Verification items for the finished model (mm, model axes). Face numbers are marked on the shaded views. A direction names the side the tool comes from. Give positions to 0.01 mm unless a question says otherwise; leave off trailing zeros. Loops run counter-clockwise (first coordinate to the right, second up) from the corner with the lowest first, then second, coordinate; pieces in that order, holes last. Notation, with made-up numbers: M 18,75.25 L 28,75.25 A19 ccw 28,85.25 Z; hole C 88,-10 d1. An arc over 180 degrees is marked long. Answer in a Markdown table with one row per item.
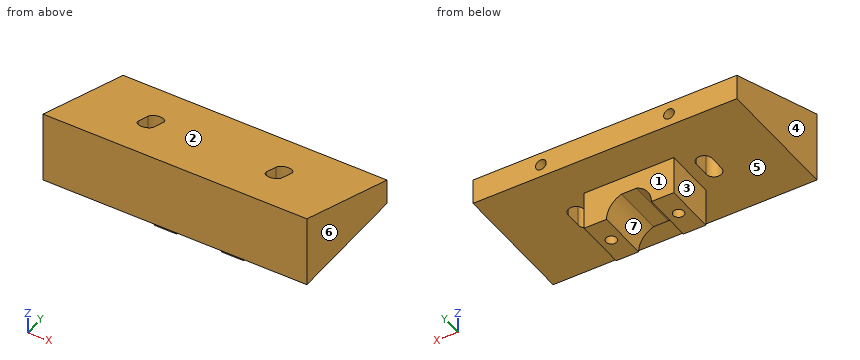
Autodesk Inventor part; units mm, degrees
ref_plane "YZ Plane" through (0, 0, 0) normal (1, 0, 0) x (0, 1, 0)
ref_plane "XZ Plane" through (0, 0, 0) normal (0, 1, 0) x (-1, 0, 0)
ref_plane "XY Plane" through (0, 0, 0) normal (0, 0, 1) x (1, 0, 0)
sketch "Skizze1" plane through (0, 0, 0) normal (0, 1, 0) x (-1, 0, 0)
  line L0 (0, 0) -> (-206, 0)
  line L1 (-206, 0) -> (-206, -20)
  line L2 (-206, -20) -> (0, -20)
  line L3 (0, -20) -> (0, 0)
  dimension "d0" = 206
  dimension "d1" = 20
extrude "Extrusion1" add sketch "Skizze1" against normal blind 100
sketch "Skizze2" plane through (0, 0, 0) normal (0, 1, 0) x (1, 0, 0)
  line L0 (0, 0) -> (0, 10) construction
  line L1 (0, 10) -> (206, 10) construction
  line L2 (0, 10) -> (103, 10) construction
  line L3 (103, 10) -> (53, 10) construction
  line L4 (53, 10) -> (153, 10) construction
  dimension "d4" = 10
  dimension "d5" = 206
  dimension "d6" = 90
  dimension "d7" = 103
  dimension "d8" = 50
  dimension "d9" = 100
hole "Bohrung1" at (153, 0, -10) at (53, 0, -10) direction (0, -1, 0) diameter 8.376 depth 27.3 tip angle 118
sketch "Skizze3" plane through (206, 0, 0) normal (1, 0, 0) x (0, 0, -1)
  line L0 (0, 0) -> (-41.0424, -112.7631)
  line L1 (0, 0) -> (120, 0) construction
  line L2 (0, 0) -> (0, -100)
  line L3 (0, -100) -> (-50, -100)
  line L4 (0, -100) -> (50, -100) construction
  point P0 (-36.397, -100)
  dimension "d17" = 120
  dimension "d18" = 110
  dimension "d19" = 50
  dimension "d20" = 180
extrude "Extrusion2" add sketch "Skizze3" against normal blind 206
sketch "Skizze4" plane through (206, 0, -20) normal (0, 0, -1) x (-1, 0, 0)
  line L0 (206, 0) -> (103, 0) construction
  line L1 (206, 0) -> (309, 0) construction
  line L2 (103, 0) -> (153, 0) construction
  line L3 (0, 0) -> (206, 0) construction
  line L4 (153, 0) -> (53, 0) construction
  line L5 (53, 0) -> (53, -50) construction
  line L6 (53, 0) -> (103, 0) construction
  line L7 (153, 0) -> (153, -50) construction
  line L8 (153, 0) -> (203, 0) construction
  line L9 (53, -50) -> (59, -50)
  line L10 (59, -50) -> (59, -44)
  arc A0 (59, -44) -> (47, -44) centre (53, -44) ccw
  line L11 (53, -44) -> (47, -44) construction
  line L12 (53, -44) -> (59, -44) construction
  line L13 (47, -44) -> (47, -50)
  line L14 (47, -50) -> (59, -50) construction
  line L15 (53, -100) -> (53, -50) construction
  line L16 (59, -50) -> (59, -56)
  arc A1 (47, -56) -> (59, -56) centre (53, -56) ccw
  line L17 (53, -56) -> (47, -56) construction
  line L18 (53, -56) -> (59, -56) construction
  line L19 (47, -56) -> (47, -50)
  line L20 (103, 0) -> (103, -100) construction
  line L21 (103, 0) -> (203, 0) construction
  line L22 (153, -50) -> (147, -50)
  line L23 (147, -50) -> (147, -44)
  arc A2 (159, -44) -> (147, -44) centre (153, -44) ccw
  line L24 (153, -44) -> (159, -44) construction
  line L25 (153, -44) -> (147, -44) construction
  line L26 (159, -44) -> (159, -50)
  line L27 (159, -50) -> (147, -50) construction
  line L28 (147, -50) -> (147, -56)
  line L29 (153, -56) -> (147, -56) construction
  line L30 (153, -56) -> (159, -56) construction
  line L31 (159, -56) -> (159, -50)
  arc A3 (147, -56) -> (159, -56) centre (153, -56) ccw
  dimension "d23" = 103
  dimension "d24" = 180
  dimension "d25" = 50
  dimension "d26" = 100
  dimension "d27" = 0
  dimension "d28" = 50
  dimension "d29" = 90
  dimension "d30" = 50
  dimension "d31" = 90
  dimension "d32" = 6
  dimension "d33" = 6
  dimension "d34" = 180
  dimension "d35" = 100
  dimension "d36" = 90
extrude "Extrusion3" cut sketch "Skizze4" against normal blind 100
sketch "Skizze5" plane through (206, 0, -20) normal (0, 0, -1) x (-1, 0, 0)
  line L0 (206, 0) -> (0, 0)
  line L1 (103, 0) -> (103, -100)
  line L2 (206, -100) -> (0, -100)
  line L3 (0, 0) -> (0, -100)
  line L4 (0, -50) -> (206, -50)
  line L5 (206, 0) -> (206, -100)
  line L6 (103, -50) -> (68, -50)
  line L7 (68, -50) -> (68, -30)
  line L8 (68, -30) -> (103, -30)
  line L9 (103, -30) -> (103, -50)
  line L10 (103, -50) -> (138, -50)
  line L11 (138, -50) -> (138, -30)
  line L12 (138, -30) -> (103, -30)
  line L13 (68, -50) -> (68, -70)
  line L14 (68, -70) -> (103, -70)
  line L15 (103, -70) -> (103, -50)
  line L16 (138, -50) -> (138, -70)
  line L17 (138, -70) -> (103, -70)
  dimension "d39" = 35
  dimension "d40" = 20
extrude "Extrusion4" add sketch "Skizze5" along normal blind 30 contours L12 L11 L4 L1 | L1 L4 L7 L8 | L16 L17 L1 L4 | L1 L14 L13 L4
sketch "Skizze6" plane through (68, -30, -20) normal (0, 1, 0) x (1, 0, 0)
  line L0 (70, 30) -> (0, 30)
  circle A0 centre (35, 30) radius 17.5
  point P0 (-68, -20)
  dimension "d43" = 35
extrude "Extrusion5" cut sketch "Skizze6" against normal blind 40
sketch "Skizze7" plane through (68, -30, -20) normal (0, 1, 0) x (1, 0, 0)
  arc A0 (17.5, 30) -> (52.5, 30) centre (35, 30) ccw
  line L0 (35, 12.5) -> (35, 13.5)
  line L1 (35, 12.5) -> (36, 12.5) construction
  line L2 (35, 13.5) -> (45, 13.5)
  line L3 (45, 13.5) -> (25, 13.5)
  point P0 (-68, -20)
  point P1 (35, 13.5)
  point P2 (29.169, 13.5)
  point P3 (40.831, 13.5)
  dimension "d46" = 1
  dimension "d47" = 90
  dimension "d48" = 10
  dimension "d49" = 90
  dimension "d50" = 20
  dimension "d51" = 0
extrude "Extrusion6" add sketch "Skizze7" against normal blind 40
sketch "Skizze8" plane through (206, 0, -50) normal (0, 0, -1) x (-1, 0, 0)
  line L0 (68, -30) -> (138, -30) construction
  line L1 (85.5, -70) -> (85.5, -30) construction
  line L2 (68, -30) -> (85.5, -70) construction
  line L3 (138, -70) -> (68, -70) construction
  line L4 (68, -70) -> (85.5, -30) construction
  line L5 (103, -30) -> (103, -70) construction
  line L6 (120.5, -70) -> (120.5, -30) construction
  line L7 (138, -30) -> (120.5, -70) construction
  line L8 (138, -70) -> (120.5, -30) construction
  point P0 (206, 0)
  point P1 (76.75, -50)
  point P2 (129.25, -50)
hole "Bohrung2" at (129.25, -50, -50) at (76.75, -50, -50) direction (0, 0, 1) diameter 8.376 depth 27.3 tip angle 118
properties part number "Motorhalterung_BT2.1"
Item 1: Sectioned sample at D-D (y = -73.5). Record the cut outline in (x, z).
Reported:
| item | result |
|---|---|
| outline | M 0,-20 L 206,-20 L 206,26.75 L 0,26.75 Z |
Item 2: Release check for a two-part mould opening along X. For the marked faces 4, 5, 6 and 7 record: released by +X, released by -X, zero draft, split by the parting line, or undercut.
Reported:
| item | result |
|---|---|
| face 4 | released by -X |
| face 5 | zero draft |
| face 6 | released by +X |
| face 7 | undercut |
Item 3: Sectioned sample at B-B (y = -21). Record the cut outline in (x, z).
Reported:
| item | result |
|---|---|
| outline | M 0,-20 L 206,-20 L 206,7.64 L 0,7.64 Z; hole C 53,-10 d8.38; hole C 153,-10 d8.38 |
Item 4: Sectioned sample at C-C (x = 18.5). Record the cut outline in (y, z), and give its area (3 significant figures).
Reported:
| item | result |
|---|---|
| outline | M -100,-20 L 0,-20 L 0,0 L -100,36.4 Z |
| area | 3,820 mm^2 |
Item 5: Tool access check on the marked faces 1, 2 and 3. Record the directions out of +Z, -Z, +X, -X, +Y, -Y that give a thin tool (end or side, any length) a straight path to the whole face; none if there is none.
Reported:
| item | result |
|---|---|
| face 1 | -Z, +X, -X, +Y |
| face 2 | +Z, +X, -X, +Y |
| face 3 | -Z, -X, +Y, -Y |
Item 6: Sectioned sample at A-A (y = -34.5). Record the cut outline in (x, z).
Reported:
| item | result |
|---|---|
| outline | M 0,-20 L 68,-20 L 68,-50 L 85.5,-50 A17.5 cw 97.17,-33.5 L 108.83,-33.5 A17.5 cw 120.5,-50 L 138,-50 L 138,-20 L 206,-20 L 206,12.56 L 0,12.56 Z |
Item 7: Go/stop test with flat-tipped pins: pin 1 (3 mm diameter, centred on x = 62.5, y = -64, fed in from -Z); pin 2 (2 mm diameter, centred on x = 114, z = -31.5, fed in from +Y); pin 3 (13.5 mm diameter, centred on x = 76.75, y = -50, fed in from -Z); pin 4 (24 mm diameter, centred on y = -42.5, z = -34.5, fed in from +X). Record where each tip stops, or that it passes through.
Reported:
| item | result |
|---|---|
| pin 1 | stops at z = -20 |
| pin 2 | stops at y = -30 |
| pin 3 | stops at z = -50 |
| pin 4 | stops at x = 138 |
Item 8: Scan lines: L1, parallel to X at y = -50, z = -30.5; L2, parallel to X at y = -46, z = -2; L3, parallel to Y at x = 76.75, z = -30.5. Record each from-to range of solid material in increasing order. Write a range as [from, to].
Reported:
| item | result |
|---|---|
| L1 | x = [68, 72.56], [80.94, 125.06], [133.44, 138] |
| L2 | x = [0, 47], [59, 147], [159, 206] |
| L3 | y = [-70, -54.19], [-45.81, -30] |
